Input: dimensioned drawing with shaded views. Units: mm. Origin: part minimum x, y, z. A direction names the side the tool comes from. Round coordinates to 2 decimals unless told otherwise and drop trailing zeros. Write each loop counter-clockwise with the first axis right and the second up, starting at its lowest first coordinate (ties: lowest second). Pieces come first, ordered by that corner, then holes. Notation, with made-up numbers: (-3.75, 79) - (12.25, 79) arc R17 cw to (12.25, 108) - close; hole circle Ø8 at (-30.5, 63.5). An arc over 180 degrees is marked (long way). Use one line per item in the form item = value.
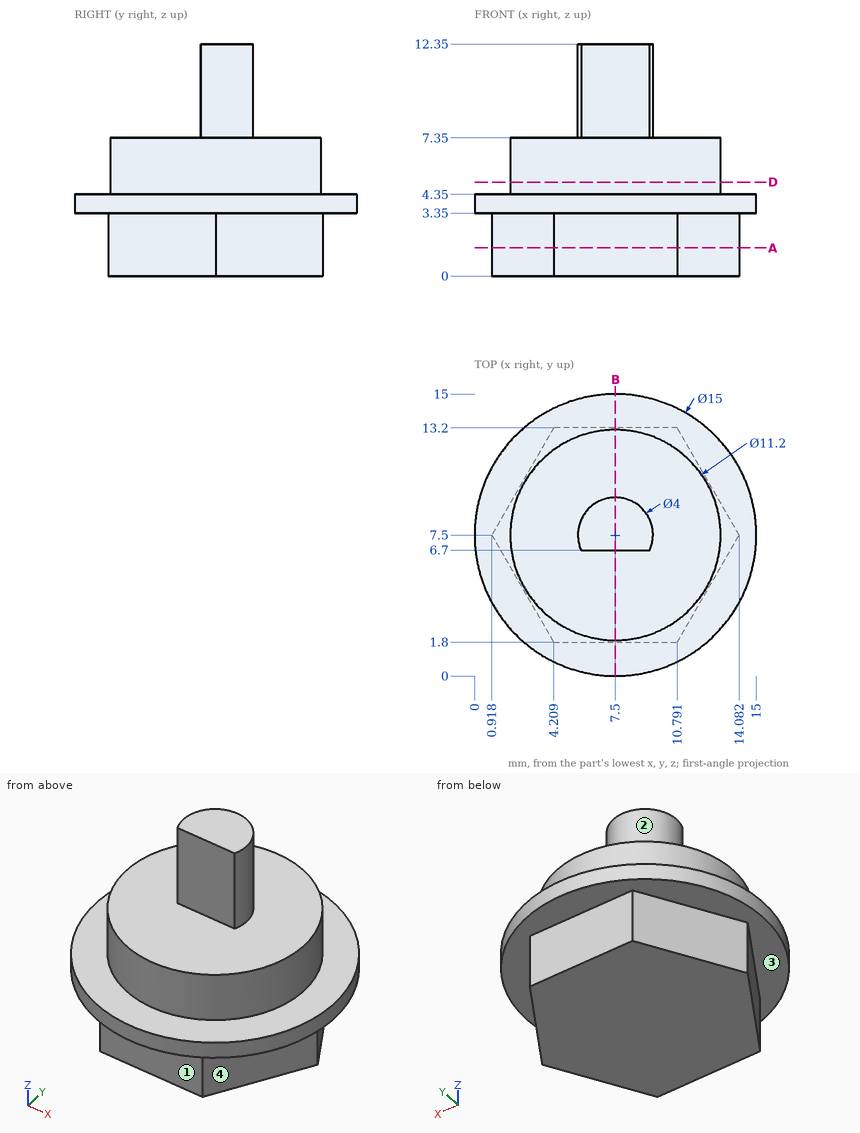
(1) First-contact query: pin 1 Ø1.5 at (x, y) = (6, 5) entering from +Z; pin 2 Ø1.8 at (x, z) = (7.5, 10) entering from -Y; pin 3 Ø1 at (x, z) = (11.5, 6.5) entering from -Y. Flat tips, straight axial feed; report the tip coordinate or a pass-through.
Derived:
pin_1 = 7.35
pin_2 = 6.7
pin_3 = 3.13
(2) Access query for the marked faces 1, 2, 3 and 4. Directions: +Z, -Z, +X, -X, +Y, -Y. A direction counts if a zero-diameter tool reaches every point of the face in a straight line with its end or side. Return the directions, or none.
Derived:
face_1 = -Z, +X, -X, -Y
face_2 = +Z
face_3 = -Z
face_4 = -Z, +X, -Y
(3) Material intervals for L1, parallel to Z at x = 4.25, y = 2.5; L2, parallel to Z at x = 7.25, y = 1.25; L3, parallel to Y at x = 10.75, z = 2.75, sorted ascending.
Derived:
L1 = 0 to 4.35
L2 = 3.35 to 4.35
L3 = 1.8 to 13.2
(4) Cut plane A-A on z = 1.5. Output: boundary loops of the cut face in (x, y), then the cut area to 3 significant figures.
Derived:
outline = (0.92, 7.5) - (4.21, 1.8) - (10.79, 1.8) - (14.08, 7.5) - (10.79, 13.2) - (4.21, 13.2) - close
area = 113 mm^2
(5) Cut plane B-B on x = 7.5. Output: boundary loops of the cut face in (y, z), then the cut area to 3 significant figures.
Derived:
outline = (0, 3.35) - (1.8, 3.35) - (1.8, 0) - (13.2, 0) - (13.2, 3.35) - (15, 3.35) - (15, 4.35) - (13.1, 4.35) - (13.1, 7.35) - (9.5, 7.35) - (9.5, 12.35) - (6.7, 12.35) - (6.7, 7.35) - (1.9, 7.35) - (1.9, 4.35) - (0, 4.35) - close
area = 101 mm^2
(6) Cut plane D-D on z = 5. Output: boundary loops of the cut face in (x, y).
Derived:
outline = circle Ø11.2 at (7.5, 7.5)
